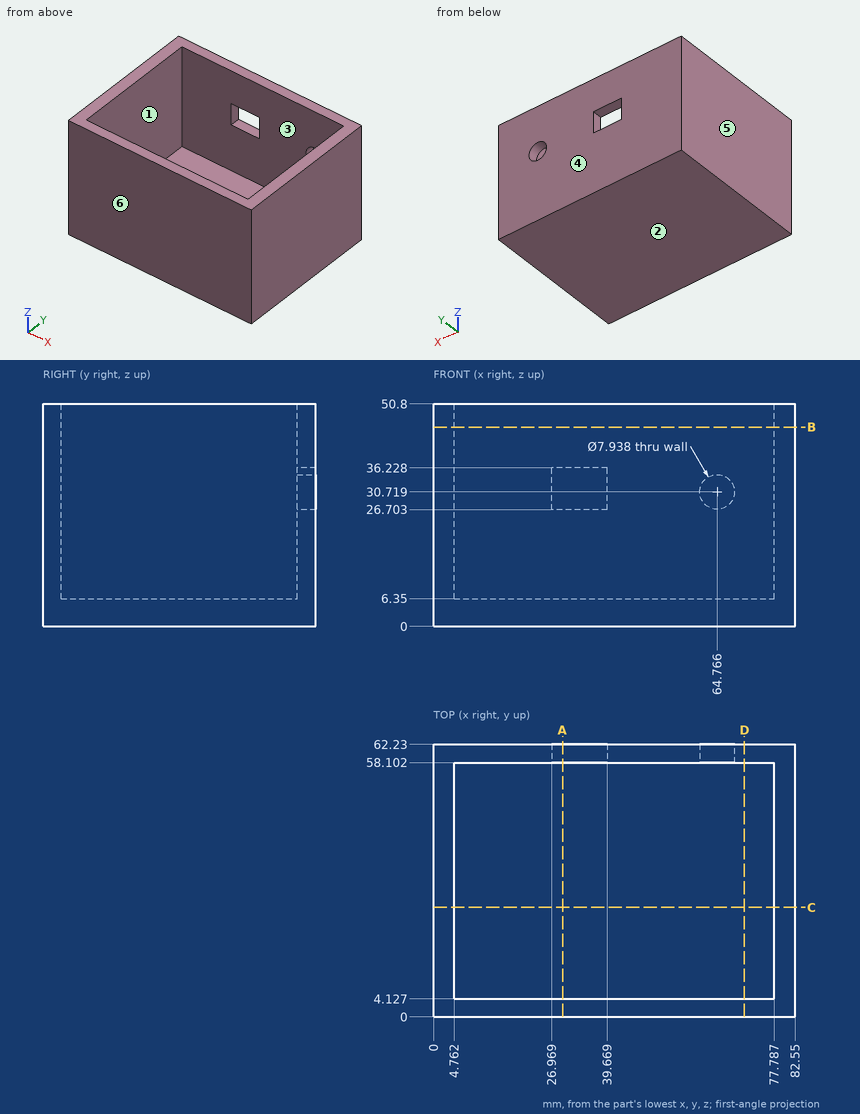
Input: dimensioned drawing with shaded views. Units: mm. Origin: part minimum x, y, z. A direction names the side the tool comes from. Coordinates: 2 decimals unless noted, no trailing zeros. Loops run counter-clockwise (first coordinate to the right, second up) from the corner with the lowest first, then second, coordinate; pieces in that order, holes last. Notation, with made-up numbers: M 27,-29.5 L 67,-29.5 A20 cw 67,8.5 Z; hole C 28.5,58 d2. An arc over 180 degrees is marked long. Use a Markdown table: item, result. Add a question column.
1) Section D-D, the plane x = 71. Return the cut outline in (y, z), plus the area to 3 significant figures.
2) Line query: L1, parallel to X at y = 20, z = 13; L2, parallel to Y at x = 59.5, z = 16; L3, parallel to Z at x = 60.5, y = 7. Output: solid intervals per line, ascending. Write a range as from..to.
3) Section C-C, the plane y = 25. Return the cut outline in (x, z).
4) Pin query (flat end, axial travel): P1, Ø10.5, axis at x = 64.77, z = 30.72, coming from the +Y side; P2, Ø4, axis at x = 44.5, y = 22.5, coming from the +Z side. Return the tip coordinate at first contact, or that it passes through.
5) Draft query along Y for the marked faces 3, 4, 5 and 6. Return one class per face: +Y half, -Y half, draft (parallel to the pull), parting line (faces both ways), or undercut.
6) Section A-A, the plane x = 29.5. Return the cut outline in (y, z).
7) Set-up query: the marked faces 1 and 2. Return all of +Z, -Z, +X, -X, +Y, -Y with unobstructed straight access to the full face (end or side cutting, diameter ignored); none if empty.
8) Section B-B, the plane z = 45.5. Return the cut outline in (x, y), plus the area to 3 significant figures.
Answer below:
| question | item | result |
|---|---|---|
| 1 | outline | M 0,0 L 62.23,0 L 62.23,50.8 L 58.1,50.8 L 58.1,6.35 L 4.13,6.35 L 4.13,50.8 L 0,50.8 Z |
| 1 | area | 762 mm2 |
| 2 | L1 | 0..4.76, 77.79..82.55 |
| 2 | L2 | 0..4.13, 58.1..62.23 |
| 2 | L3 | 0..6.35 |
| 3 | outline | M 0,0 L 82.55,0 L 82.55,50.8 L 77.79,50.8 L 77.79,6.35 L 4.76,6.35 L 4.76,50.8 L 0,50.8 Z |
| 4 | P1 | y = 62.23 |
| 4 | P2 | z = 6.35 |
| 5 | face 3 | undercut |
| 5 | face 4 | +Y half |
| 5 | face 5 | draft |
| 5 | face 6 | -Y half |
| 6 | outline | M 0,0 L 62.23,0 L 62.23,26.7 L 58.1,26.7 L 58.1,6.35 L 4.13,6.35 L 4.13,50.8 L 0,50.8 Z; M 58.1,36.23 L 62.23,36.23 L 62.23,50.8 L 58.1,50.8 Z |
| 7 | face 1 | +Z |
| 7 | face 2 | -Z, +X, -X, +Y, -Y |
| 8 | outline | M 0,0 L 82.55,0 L 82.55,62.23 L 0,62.23 Z; hole M 4.76,4.13 L 77.79,4.13 L 77.79,58.1 L 4.76,58.1 Z |
| 8 | area | 1,200 mm2 |
